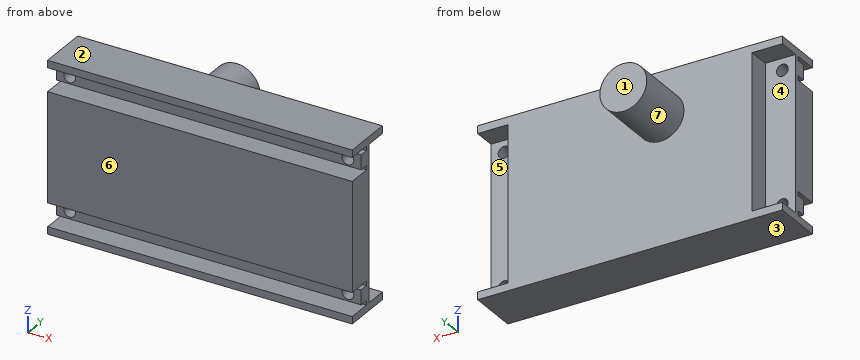
from build123d import *

# Parameters (mm, degrees)
SKETCH1_W             = 104
SKETCH1_H             = 58.2
BOSS_EXTRUDE1_DEPTH   = 17
CUT_EXTRUDE2_DEPTH    = 105
SKETCH3_R             = 8
BOSS_EXTRUDE2_DEPTH   = 21
F_4_0MM_DOWEL_HOLE1_D = 4
SKETCH6_W             = 53
SKETCH6_H             = 7.475
CUT_EXTRUDE3_DEPTH    = 10.31875


with BuildPart() as part:
    # Sketch1 → Boss-Extrude1 (new body)
    with BuildSketch(Plane(origin=(0, 0, 0), x_dir=(1, 0, 0), z_dir=(0, 1, 0))):
        with Locations((52, 29.1)):
            Rectangle(SKETCH1_W, SKETCH1_H)
    extrude(amount=BOSS_EXTRUDE1_DEPTH)

    # Sketch2 → Cut-Extrude2 (cut, through all)
    with BuildSketch(Plane(origin=(104, 0, 0), x_dir=(0, 0, -1), z_dir=(1, 0, 0))):
        Polygon((2.5, 0), (2.5, 8), (4, 8), (4, 5), (9, 5), (9, 8), (10.5, 8), (10.5, 0), align=None)
        Polygon((47.7, 8), (47.7, 0), (55.7, 0), (55.7, 8), (54.2, 8), (54.2, 5), (49.2, 5), (49.2, 8), align=None)
    extrude(amount=-CUT_EXTRUDE2_DEPTH, mode=Mode.SUBTRACT)

    # Sketch3 → Boss-Extrude2 (add)
    with BuildSketch(Plane(origin=(0, 17, 0), x_dir=(1, 0, 0), z_dir=(0, 1, 0))):
        with Locations((41.573485345, 15.236601424)):
            Circle(SKETCH3_R)
    extrude(amount=BOSS_EXTRUDE2_DEPTH)

    # Ø4.0mm Dowel Hole1 (through all)
    with Locations(Plane(origin=(0, 5, 0), x_dir=(-1, 0, 0), z_dir=(0, -1, 0))):
        with Locations((-4.5, 51.6), (-4.5, 6.6), (-99.5, 6.6), (-99.5, 51.6)):
            Hole(F_4_0MM_DOWEL_HOLE1_D / 2)

    # Sketch6 → Cut-Extrude3 (cut)
    with BuildSketch(Plane(origin=(104, 0, 0), x_dir=(0, 0, -1), z_dir=(1, 0, 0))):
        with Locations((29.1, 13.2625)):
            Rectangle(SKETCH6_W, SKETCH6_H)
    cut_extrude3 = extrude(amount=-CUT_EXTRUDE3_DEPTH, mode=Mode.SUBTRACT)

    # Mirror1: Cut-Extrude3 across plane
    add(cut_extrude3.mirror(Plane.ZY.offset(-52.00000014)), mode=Mode.SUBTRACT)


solid = part.part
Input: part model. Units: mm. Frame: model coordinates. Face numbers are marked on the shaded views. A direction names the side the tool comes from. Give positions to 0.01 mm unless a question says otherwise; leave off trailing zeros. Loops run counter-clockwise (first coordinate to the right, second up) from the corner with the lowest first, then second, coordinate; pieces in that order, holes last. Notation, with made-up numbers: M 88.25,78.25 L 111.25,78.25 A14 cw 111.25,93.25 Z; hole C 67.25,-2.5 d7. An arc over 180 degrees is marked long. Use CSV: the item, a comma, the result in double quotes.
(1) Pin query (flat end, axial travel): P1, Ø4, axis at y = 15, z = -13, coming from the -X side; P2, Ø5, axis at x = 99.5, z = -51.6, coming from the -Y side; P3, Ø3, axis at x = 2.5, z = -20, coming from the +Y side (3 decimals). Return the tip coordinate at first contact, or that it passes through.
Outcome:
P1,"stops at x = 10.32"
P2,"stops at y = 5"
P3,"stops at y = 9.525"
(2) Section A-A, the plane x = 99.5. Count the separate pieces of the cut face and the enclosed holes in it, plus the area to 3 significant figures.
Outcome:
separate pieces,"3"
enclosed holes,"0"
area,"459 mm²"
(3) Pull-direction query (Z, two-part tool) for the marked faces 1, 2, 3 and 4; classes: pulls with the +Z half, pulls with the -Z half, needs draft (parallel to the pull), parting line crosses it, or undercut.
Outcome:
face 1,"needs draft"
face 2,"pulls with the +Z half"
face 3,"pulls with the -Z half"
face 4,"undercut"
(4) Section D-D, the plane x = 61. Return loops of the section in (y, z).
Outcome:
outline,"M 0,-58.2 L 17,-58.2 L 17,0 L 0,0 L 0,-2.5 L 8,-2.5 L 8,-4 L 5,-4 L 5,-9 L 8,-9 L 8,-10.5 L 0,-10.5 L 0,-47.7 L 8,-47.7 L 8,-49.2 L 5,-49.2 L 5,-54.2 L 8,-54.2 L 8,-55.7 L 0,-55.7 Z"
(5) Material intervals for L1, parallel to Z at x = 88.5, y = 5.5; L2, parallel to Z at x = 27, y = 3; L3, parallel to Y at x = 61, z = -48, sorted ascending. Write a range as [from, to].
Outcome:
L1,"z = [-58.2, -55.7], [-54.2, -49.2], [-47.7, -10.5], [-9, -4], [-2.5, 0]"
L2,"z = [-58.2, -55.7], [-47.7, -10.5], [-2.5, 0]"
L3,"y = [8, 17]"
(6) Section C-C, the plane z = -27. Return loops of the section in (x, y) (3 decimals), plus the area to 3 significant figures.
Outcome:
outline,"M 0,0 L 104,0 L 104,9.525 L 93.681,9.525 L 93.681,17 L 10.319,17 L 10.319,9.525 L 0,9.525 Z"
area,"1,610 mm²"
(7) Section B-B, the plane z = -51.6. Return loops of the section in (x, y) (3 decimals), plus the area to 3 significant figures.
Outcome:
outline,"M 0,5 L 2.5,5 L 2.5,9.525 L 0,9.525 Z; M 6.5,5 L 97.5,5 L 97.5,9.525 L 93.681,9.525 L 93.681,17 L 10.319,17 L 10.319,9.525 L 6.5,9.525 Z; M 101.5,5 L 104,5 L 104,9.525 L 101.5,9.525 Z"
area,"1,060 mm²"
(8) Set-up query: the marked faces 5, 6 and 7. Return all of +Z, -Z, +X, -X, +Y, -Y with unobstructed straight access to the full face (end or side cutting, diameter ignored); none if empty.
Outcome:
face 5,"+X, +Y"
face 6,"+Z, -Z, +X, -X, -Y"
face 7,"+Y"
